```python
from build123d import *

# Parameters (mm, degrees)
SKETCH1_W           = 64
SKETCH1_H           = 38.5
BOSS_EXTRUDE1_DEPTH = 26
SKETCH2_W           = 58
SKETCH2_H           = 35
CUT_EXTRUDE1_DEPTH  = 17
SKETCH4_W           = 45
SKETCH4_H           = 35
CUT_EXTRUDE3_DEPTH  = 7
SKETCH5_R           = 6.375
CUT_EXTRUDE4_DEPTH  = 12
SKETCH6_W           = 9.989337028
SKETCH6_H           = 24.5
CUT_EXTRUDE5_DEPTH  = 17
SKETCH7_R           = 3.375
CUT_EXTRUDE6_DEPTH  = 7
SKETCH8_W           = 9
SKETCH8_H           = 4
CUT_EXTRUDE7_DEPTH  = 7
FILLET1_R           = 2.5
SKETCH10_W          = 59.5
SKETCH10_H          = 0.75
CUT_EXTRUDE8_DEPTH  = 1
SKETCH11_W          = 59.75
SKETCH11_H          = 0.75
CUT_EXTRUDE9_DEPTH  = 1
SKETCH12_W          = 1
SKETCH12_H          = 36.5
SKETCH12_W_2        = 0.75
CUT_EXTRUDE10_DEPTH = 1
SKETCH13_W          = 4
SKETCH13_H          = 0.45
CUT_EXTRUDE11_DEPTH = 0.45
FILLET2_R           = 0.4
SKETCH14_W          = 4
SKETCH14_H          = 0.45
CUT_EXTRUDE12_DEPTH = 0.45
FILLET3_R           = 0.4


with BuildPart() as part:
    # Sketch1 → Boss-Extrude1 (new body)
    with BuildSketch(Plane.XY):
        with Locations((32, 19.25)):
            Rectangle(SKETCH1_W, SKETCH1_H)
    extrude(amount=BOSS_EXTRUDE1_DEPTH)

    # Sketch2 → Cut-Extrude1 (cut)
    with BuildSketch(Plane.XY.offset(26)):
        with Locations((31, 19.5)):
            Rectangle(SKETCH2_W, SKETCH2_H)
    extrude(amount=-CUT_EXTRUDE1_DEPTH, mode=Mode.SUBTRACT)

    # Sketch4 → Cut-Extrude3 (cut)
    with BuildSketch(Plane.XY.offset(9)):
        with Locations((31, 19.5)):
            Rectangle(SKETCH4_W, SKETCH4_H)
    extrude(amount=-CUT_EXTRUDE3_DEPTH, mode=Mode.SUBTRACT)

    # Sketch5 → Cut-Extrude4 (cut)
    with BuildSketch(Plane(origin=(0, 0, 0), x_dir=(-1, 0, 0), z_dir=(0, 0, -1))):
        with Locations((-56, 19.5)):
            Circle(SKETCH5_R)
        with Locations((-10.002659036, 19.005404936)):
            Circle(SKETCH5_R)
    extrude(amount=-CUT_EXTRUDE4_DEPTH, mode=Mode.SUBTRACT)

    # Sketch6 → Cut-Extrude5 (cut)
    with BuildSketch(Plane(origin=(64, 0, 0), x_dir=(0, 0, -1), z_dir=(1, 0, 0))):
        with Locations((-15.005331486, 23.25)):
            Rectangle(SKETCH6_W, SKETCH6_H)
    extrude(amount=-CUT_EXTRUDE5_DEPTH, mode=Mode.SUBTRACT)

    # Sketch7 → Cut-Extrude6 (cut)
    with BuildSketch(Plane.ZY):
        with Locations((18, 7.5)):
            Circle(SKETCH7_R)
    extrude(amount=-CUT_EXTRUDE6_DEPTH, mode=Mode.SUBTRACT)

    # Sketch8 → Cut-Extrude7 (cut)
    with BuildSketch(Plane.XZ):
        with Locations((32.5, 17)):
            Rectangle(SKETCH8_W, SKETCH8_H)
    extrude(amount=-CUT_EXTRUDE7_DEPTH, mode=Mode.SUBTRACT)

    # Fillet1
    fillet1_edges = [part.edges().sort_by_distance(p)[0] for p in [
        (0, 38.5, 13),
        (64, 38.5, 13),
        (64, 0, 13),
        (0, 0, 13),
    ]]
    fillet(fillet1_edges, radius=FILLET1_R)

    # Sketch10 → Cut-Extrude8 (cut)
    with BuildSketch(Plane.XY.offset(26)):
        with Locations((31.25, 37.375)):
            Rectangle(SKETCH10_W, SKETCH10_H)
    extrude(amount=-CUT_EXTRUDE8_DEPTH, mode=Mode.SUBTRACT)

    # Sketch11 → Cut-Extrude9 (cut)
    with BuildSketch(Plane.XY.offset(26)):
        with Locations((31.125, 1.625)):
            Rectangle(SKETCH11_W, SKETCH11_H)
    extrude(amount=-CUT_EXTRUDE9_DEPTH, mode=Mode.SUBTRACT)

    # Sketch12 → Cut-Extrude10 (cut)
    with BuildSketch(Plane.XY.offset(26)):
        with Locations((60.5, 19.5)):
            Rectangle(SKETCH12_W, SKETCH12_H)
        with Locations((1.625, 19.5)):
            Rectangle(SKETCH12_W_2, SKETCH12_H)
    extrude(amount=-CUT_EXTRUDE10_DEPTH, mode=Mode.SUBTRACT)

    # Sketch13 → Cut-Extrude11 (cut)
    with BuildSketch(Plane(origin=(0, 1.25, 0), x_dir=(1, 0, 0), z_dir=(0, 1, 0))):
        with Locations((29.75, -25.475)):
            Rectangle(SKETCH13_W, SKETCH13_H)
        with Locations((22.75, -25.475)):
            Rectangle(SKETCH13_W, SKETCH13_H)
        with Locations((36.75, -25.475)):
            Rectangle(SKETCH13_W, SKETCH13_H)
    extrude(amount=-CUT_EXTRUDE11_DEPTH, mode=Mode.SUBTRACT)

    # Fillet2
    # the kernel refuses this fillet: 0.4 mm, written as the material it takes off along each edge
    with BuildSketch(Plane(origin=(34.75, 1.25, 25.25), x_dir=(0, 0, -1), z_dir=(1, 0, 0)), Plane(origin=(20.75, 1.25, 25.25), x_dir=(0, 0, -1), z_dir=(1, 0, 0)), Plane(origin=(27.75, 1.25, 25.25), x_dir=(0, 0, -1), z_dir=(1, 0, 0))) as fillet2_piece_1:
        with BuildLine():
            CenterArc((0.4, -0.370809924), FILLET2_R, 112.024312837, 67.975687163)
            Line((0, -0.370809924), (0, 0))
            Line((0, 0), (0.25, 0))
        make_face()
    extrude(amount=4, mode=Mode.SUBTRACT)
    with BuildSketch(Plane(origin=(38.75, 1.25, 25.7), x_dir=(0, 0, 1), z_dir=(-1, 0, 0)), Plane(origin=(24.75, 1.25, 25.7), x_dir=(0, 0, 1), z_dir=(-1, 0, 0)), Plane(origin=(31.75, 1.25, 25.7), x_dir=(0, 0, 1), z_dir=(-1, 0, 0))) as fillet2_piece_2:
        with BuildLine():
            CenterArc((FILLET2_R, -FILLET2_R), FILLET2_R, 90, 90)
            Line((0, -FILLET2_R), (0, 0))
            Line((0, 0), (FILLET2_R, 0))
        make_face()
    extrude(amount=4, mode=Mode.SUBTRACT)

    # Sketch14 → Cut-Extrude12 (cut)
    with BuildSketch(Plane.XZ.offset(-37.75)):
        with Locations((29.75, 25.475)):
            Rectangle(SKETCH14_W, SKETCH14_H)
        with Locations((36.75, 25.475)):
            Rectangle(SKETCH14_W, SKETCH14_H)
        with Locations((22.75, 25.475)):
            Rectangle(SKETCH14_W, SKETCH14_H)
    extrude(amount=-CUT_EXTRUDE12_DEPTH, mode=Mode.SUBTRACT)

    # Fillet3
    # the kernel refuses this fillet: 0.4 mm, written as the material it takes off along each edge
    with BuildSketch(Plane(origin=(24.75, 37.75, 25.7), x_dir=(0, 0, 1), z_dir=(-1, 0, 0))) as fillet3_piece_1:
        with BuildLine():
            CenterArc((FILLET3_R, FILLET3_R), FILLET3_R, 180, 90)
            Line((0, FILLET3_R), (0, 0))
            Line((0, 0), (FILLET3_R, 0))
        make_face()
    extrude(amount=4, mode=Mode.SUBTRACT)
    with BuildSketch(Plane(origin=(20.75, 37.75, 25.25), x_dir=(0, 0, -1), z_dir=(1, 0, 0))) as fillet3_piece_2:
        with BuildLine():
            CenterArc((0.4, 0.370809924), FILLET3_R, 180, 67.975687163)
            Line((0, 0.370809924), (0, 0))
            Line((0, 0), (0.25, 0))
        make_face()
    extrude(amount=4, mode=Mode.SUBTRACT)
    with BuildSketch(Plane(origin=(38.75, 37.75, 25.25), x_dir=(0, 0, -1), z_dir=(-1, 0, 0)), Plane(origin=(31.75, 37.75, 25.25), x_dir=(0, 0, -1), z_dir=(-1, 0, 0))) as fillet3_piece_3:
        with BuildLine():
            CenterArc((0.4, -0.370809924), FILLET3_R, 112.024312837, 67.975687163)
            Line((0, -0.370809924), (0, 0))
            Line((0, 0), (0.25, 0))
        make_face()
    extrude(amount=4, mode=Mode.SUBTRACT)
    with BuildSketch(Plane(origin=(34.75, 37.75, 25.7), x_dir=(0, 0, 1), z_dir=(1, 0, 0)), Plane(origin=(27.75, 37.75, 25.7), x_dir=(0, 0, 1), z_dir=(1, 0, 0))) as fillet3_piece_4:
        with BuildLine():
            CenterArc((FILLET3_R, -FILLET3_R), FILLET3_R, 90, 90)
            Line((0, -FILLET3_R), (0, 0))
            Line((0, 0), (FILLET3_R, 0))
        make_face()
    extrude(amount=4, mode=Mode.SUBTRACT)


solid = part.part
```
The listing builds one solid part. Answer for the finished solid, in the listing's coordinates (mm). A direction names the side the tool comes from. Round coordinates to 2 decimals unless told otherwise and drop trailing zeros. Loops run counter-clockwise (first coordinate to the right, second up) from the corner with the lowest first, then second, coordinate; pieces in that order, holes last.
Q1. For a pull along Y with two mould halves and no side action, classify faces 1 (the face through (8.5, 31, 6)), 2 (the face through (32, 1, 15)), 3 (the face through (32, 0, 13)) as released by +Y, released by -Y, zero draft, split by the parting line, or undercut.
Q2. Section A-A, the plane y = 7.5 is taken. Determine the outline of the cut face in (x, z) (3 decimals), then the cut area to 3 significant figures.
Q3. Find the intervals of material crossed by line 1 (Y direction, x = 47, z = 23.5); line 2 (X direction, y = 29, z = 9.5); line 3 (Y direction, x = 56, z = 5) (3 decimals), in increasing order.
Q4. Given pin 1 Ø3 at (x, y) = (23, 14.5) entering from +Z; pin 2 Ø3 at (y, z) = (15.5, 14) entering from +X, each flat-ended and moving along its own axis, determine where each tip first touches the part or whether it passes through.
Q5. Section C-C, the plane x = 56 is taken. Determine the outline of the cut face in (y, z) (3 decimals), then the cut area to 3 significant figures.
Q6. Section B-B, the plane z = 18 is taken. Determine the outline of the cut face in (x, y) (3 decimals), then the cut area to 3 significant figures.
Q7. Which of the six approach directions +Z, -Z, +X, -X, +Y, -Y give full straight-line access (tool end or side, diameter ignored) to faces 4 (the face through (0.99, 7.65, 14.63)), 5 (the face through (62, 35.5, 15)), 6 (the face through (57, 8, 9))?
Q8. Section D-D, the plane z = 4.5 is taken. Determine the outline of the cut face in (x, y) (3 decimals), then the cut area to 3 significant figures.
Completed:
1. face 1: undercut
1. face 2: zero draft
1. face 3: released by -Y
2. outline: (0, 0) - (64, 0) - (64, 26) - (61, 26) - (61, 25) - (60, 25) - (60, 9) - (53.5, 9) - (53.5, 2) - (8.5, 2) - (8.5, 9) - (2, 9) - (2, 14.625) - (0, 14.625) - close; (0, 21.375) - (2, 21.375) - (2, 25) - (1.25, 25) - (1.25, 26) - (0, 26) - close
2. area: 348 mm2
3. line 1: y = 0 to 2, 37 to 38.5
3. line 2: x = 0 to 2, 60 to 64
3. line 3: y = 0 to 13.125, 25.875 to 38.5
4. pin 1: stops at z = 2
4. pin 2: stops at x = 2
5. outline: (0, 0) - (13.125, 0) - (13.125, 9) - (2, 9) - (2, 25) - (1.25, 25) - (1.25, 26) - (0, 26) - close; (25.875, 0) - (38.5, 0) - (38.5, 26) - (37.75, 26) - (37.75, 25) - (37, 25) - (37, 9) - (25.875, 9) - close
5. area: 290 mm2
6. outline: (0, 2.5) arc R2.5 ccw to (2.5, 0) - (28, 0) - (28, 2) - (2, 2) - (2, 4.125) - (0, 4.125) - close; (0, 10.875) - (2, 10.875) - (2, 37) - (60, 37) - (60, 35.5) - (64, 35.5) - (64, 36) arc R2.5 ccw to (61.5, 38.5) - (2.5, 38.5) arc R2.5 ccw to (0, 36) - close; (37, 0) - (61.5, 0) arc R2.5 ccw to (64, 2.5) - (64, 11) - (60, 11) - (60, 2) - (37, 2) - close
6. area: 299 mm2
7. face 4: -X
7. face 5: +X
7. face 6: +Z
8. outline: (0, 2.5) arc R2.5 ccw to (2.5, 0) - (61.5, 0) arc R2.5 ccw to (64, 2.5) - (64, 36) arc R2.5 ccw to (61.5, 38.5) - (2.5, 38.5) arc R2.5 ccw to (0, 36) - close; hole (8.5, 2) - (53.5, 2) - (53.5, 13.636) arc R6.375 ccw (long way) to (53.5, 25.364) - (53.5, 37) - (8.5, 37) - (8.5, 25.201) arc R6.375 ccw to (8.5, 12.81) - close
8. area: 744 mm2
